Autodesk Inventor part; units mm, degrees
ref_plane "YZ Plane" through (0, 0, 0) normal (1, 0, 0) x (0, 1, 0)
ref_plane "XZ Plane" through (0, 0, 0) normal (0, 1, 0) x (-1, 0, 0)
ref_plane "XY Plane" through (0, 0, 0) normal (0, 0, 1) x (1, 0, 0)
sketch "Boceto1" plane through (0, 0, 0) normal (0, 0, 1) x (1, 0, 0)
  line L0 (0, 0) -> (-500, 0)
  line L1 (0, 0) -> (500, 0)
  line L2 (0, 0) -> (0, 300)
  line L3 (-500, 0) -> (0, 300)
  line L4 (500, 0) -> (0, 300)
  dimension "d0" = 500
  dimension "d1" = 500
  dimension "d2" = 300
extrude "Extrusión1" add sketch "Boceto1" along normal blind 1000
sketch "Boceto2" plane through (-500, 0, 0) normal (0, -1, 0) x (1, 0, 0)
  line L0 (0, 1000) -> (1000, 1000)
  line L1 (0, 1000) -> (0, 800)
  line L2 (0, 0) -> (0, 1000)
  line L3 (0, 800) -> (200, 1000)
  line L4 (200, 1000) -> (0, 1000)
  line L5 (1000, 1000) -> (800, 1000)
  line L6 (800, 1000) -> (1000, 800)
  line L7 (1000, 0) -> (1000, 1000)
  line L8 (1000, 800) -> (1000, 1000)
  line L9 (0, 0) -> (1000, 0)
  line L10 (0, 0) -> (0, 200)
  line L11 (200, 0) -> (0, 0)
  line L12 (200, 0) -> (0, 200)
  line L13 (1000, 0) -> (800, 0)
  line L14 (800, 0) -> (1000, 0)
  line L15 (1000, 200) -> (800, 0)
  point P0 (500, 0)
  dimension "d5" = 200
  dimension "d6" = 45
  dimension "d7" = 200
  dimension "d8" = 45
extrude "Extrusión2" cut sketch "Boceto2" against normal blind 1000 contours L0 L3 L1 | L0 L7 L6 | L12 L9 L2 | L7 L9 L15
sketch "Boceto3" plane through (0, 300, 1000) normal (0.5145, 0.8575, 0) x (0.8575, -0.5145, 0)
  line L0 (583.0952, 800) -> (583.0952, 200)
  arc A0 (583.0952, 200) -> (583.0952, 800) centre (63.4799, 500) ccw
  line L1 (583.0952, 800) -> (473.0952, 800)
  line L2 (473.0952, 800) -> (473.0952, 200)
  line L3 (473.0952, 200) -> (583.0952, 200)
  line L4 (583.0952, 200) -> (583.0952, 800)
  point P0 (154.3487, 1000)
  dimension "d11" = 600
  dimension "d12" = 110
extrude "Extrusión3" add sketch "Boceto3" against normal blind 20
sketch "Boceto4" plane through (0, 300, 1000) normal (-0.5145, 0.8575, 0) x (0.8575, 0.5145, 0)
  line L0 (-583.0952, 800) -> (-583.0952, 200)
  arc A0 (-583.0952, 800) -> (-583.0952, 200) centre (-63.4799, 500) ccw
  line L1 (-583.0952, 800) -> (-473.0952, 800)
  line L2 (-473.0952, 800) -> (-473.0952, 200)
  line L3 (-473.0952, 200) -> (-583.0952, 200)
  line L4 (-583.0952, 200) -> (-583.0952, 800)
  point P0 (-154.3487, 1000)
  dimension "d15" = 600
  dimension "d16" = 110
extrude "Extrusión4" add sketch "Boceto4" against normal blind 20
sketch "Boceto5" plane through (0, 0, 0) normal (0, 0, -1) x (-1, 0, 0)
  line L0 (-300, 120) -> (0, 300)
  line L1 (0, 300) -> (0, 200)
  line L2 (0, 200) -> (25, 200)
  line L3 (0, 200) -> (-25, 200)
  line L4 (-25, 200) -> (-25, 600)
  line L5 (-25, 600) -> (25, 600)
  line L6 (25, 600) -> (25, 200)
  point P0 (0, 0)
  dimension "d19" = 100
  dimension "d20" = 25
  dimension "d21" = 25
  dimension "d22" = 400
extrude "Extrusión5" add sketch "Boceto5" along normal blind 200 and the other way blind 1200
sketch "Boceto6" plane through (-300, 0, 0) normal (0, -1, 0) x (1, 0, 0)
  line L0 (275, 1000) -> (275, 0)
  circle A0 centre (275, 500) radius 250
  point P0 (300, 0)
  dimension "d27" = 500
extrude "Extrusión6" add sketch "Boceto6" along normal blind 700
properties part number "Base_rotativa"
CAD build for the part. Positions are in the model's coordinates, mm. A direction names the side the tool comes from. Round coordinates to 2 decimals unless told otherwise and drop trailing zeros. Write each loop counter-clockwise with the first axis right and the second up, starting at its lowest first coordinate (ties: lowest second). Pieces come first, ordered by that corner, then holes. Notation, with made-up numbers: (83, 20) -> (121, 20) arc R7 cw to (121, 29) -> close; hole circle Ø10 at (23, 18). An arc over 180 degrees is marked (long way). Answer in a Markdown table with one row per item. Add a question column.
Item 1: Saw through at C-C, the plane y = -556. Write the cut outline in (x, z).
Item 2: Saw through at A-A, the plane z = 127. Write the cut outline in (x, y).
Item 3: Saw through at D-D, the plane z = 500. Write the cut outline in (x, y).
Item 4: Drill centre lines: line 1 (X direction, y = 314, z = 1086); line 2 (Y direction, x = 139.5, z = 591.5); line 3 (Y direction, x = 22.5, z = 1124). Where is each one in solid material? Low to high. Write a range as from..to.
Item 5: Which spindle directions (+Z, -Z, +X, -X, +Y, -Y) get a long thin tool onto all of the face, cutting with end or side? Do faces 5 (the face through (-379, 32, 921)), 6 (the face through (0, 200, 1101)), 7 (the face through (-79.195, -345.1, 744.055)), 8 (the face through (-28, -700, 504)), 9 (the face through (0, 200, -99)). Say none if no direction does.
Item 6: Mould opens along X. For faces 1 (the face through (215, 0, 382)), 2 (the face through (0, 600, 510)), 3 (the face through (-240, 156, 493)), 4 (the face through (498.366, -22.343, 495.8)) say: pulls with the +X half, pulls with the -X half, needs draft (parallel to the pull), parting line crosses it, or undercut.
Item 7: Saw through at B-B, the plane x = -125.5. Write the cut outline in (y, z).
Item 8: Drop flat-ended pins along their axis: pin 1 Ø19 at (x, y) = (481, -5.5) entering from -Z; pin 2 Ø5 at (x, y) = (489, -10) entering from +Z; pin 3 Ø1.5 at (x, z) = (-246, 138) entering from -Y. Give the stop position or say it passes through.
Findings below:
| question | item | result |
|---|---|---|
| 1 | outline | circle Ø500 at (-25, 500) |
| 2 | outline | (-427, 0) -> (427, 0) -> (427, 43.8) -> (25, 285) -> (25, 600) -> (-25, 600) -> (-25, 285) -> (-427, 43.8) -> close |
| 3 | outline | (-568.93, -41.36) -> (-558.64, -58.51) -> (-461.13, 0) -> (-275, 0) -> (-275, -700) -> (225, -700) -> (225, 0) -> (461.13, 0) -> (558.64, -58.51) -> (568.93, -41.36) -> (25, 285) -> (25, 600) -> (-25, 600) -> (-25, 285) -> close |
| 4 | line 1 | x = -25..25 |
| 4 | line 2 | y = -700..216.3 |
| 4 | line 3 | y = 200..600 |
| 5 | face 5 | +Z, -X, +Y, -Y |
| 5 | face 6 | +Z, +X, -X, -Y |
| 5 | face 7 | -Y |
| 5 | face 8 | +Z, -Z, +X, -X, -Y |
| 5 | face 9 | -Z, +X, -X, -Y |
| 6 | face 1 | undercut |
| 6 | face 2 | needs draft |
| 6 | face 3 | pulls with the -X half |
| 6 | face 4 | undercut |
| 7 | outline | (-700, 271.09) -> (0, 271.09) -> (0, 0) -> (224.7, 0) -> (224.7, 1000) -> (0, 1000) -> (0, 728.91) -> (-700, 728.91) -> close |
| 8 | pin 1 | stops at z = 173.25 |
| 8 | pin 2 | stops at z = 800 |
| 8 | pin 3 | stops at y = 0 |
